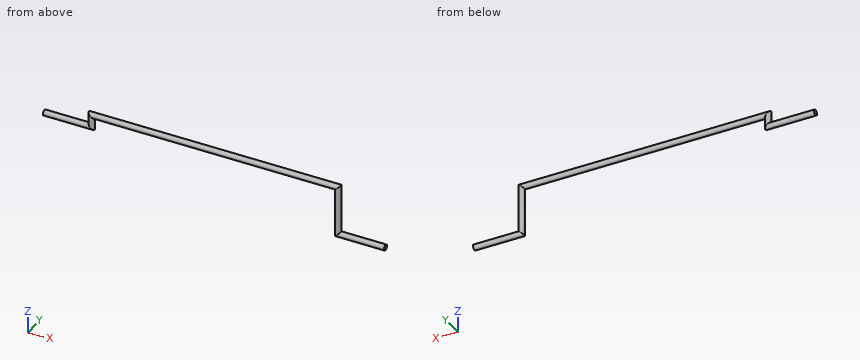
from build123d import *

# Parameters (mm, degrees)
SWEEP1_PROFILE_R = 0.6


with BuildPart() as part:
    # Sweep1: sweep along a path in Sketch1
    with BuildLine(Plane(origin=(0, 0, 0), x_dir=(1, 0, 0), z_dir=(0, 1, 0))) as sweep1_path:
        Line((62.11, 10.55), (52.11, 10.55))
        Line((52.11, 10.55), (52.11, 0))
        Line((52.11, 0), (0, 0))
        Line((0, 0), (0, 2.6))
        Line((0, 2.6), (-10, 2.6))
    # Sweep1 profile (on start of the path) → Sweep1 (sweep)
    with BuildSketch(Plane(origin=(62.11, 0, -10.55), x_dir=(0, 0, -1), z_dir=(-1, 0, 0))):
        Circle(SWEEP1_PROFILE_R)
    sweep(path=sweep1_path.line, transition=Transition.RIGHT)


solid = part.part
Check sheet for the modelled part. Datum: model origin and axes. Units: mm. Give positions to 0.01 mm unless a question says otherwise; leave off trailing zeros. Order: outer loops, then holes, each group sorted by start corner. A loop starts at its lowest first (then second) coordinate and runs counter-clockwise, first axis right, second up. Notation, with made-up numbers: (-27.75, 51.5) - (-23.75, 51.5) arc R28 ccw to (-23.75, 80.5) - close; hole circle Ø7 at (36, 61.5). An arc over 180 degrees is marked (long way). Answer as CSV lines item,"result".
1. Section check D-D (x = -5). Record the boundary of the cut face in (y, z), then the cut area to 3 significant figures.
Result sheet:
outline,"circle Ø1.2 at (0, -2.6)"
area,"1.13 mm²"
2. Section check A-A (z = -2.6). Record the boundary of the cut face in (x, y).
Result sheet:
outline,"(-10, -0.6) - (0, -0.6) arc R0.6 ccw to (0, 0.6) - (-10, 0.6) - close; circle Ø1.2 at (52.11, 0)"
3. Scan lines: probe 1 along Z at (x, y) = (39, -0.05); probe 2 along X at (y, z) = (0.4, -1.5); probe 3 along X at (y, z) = (-0.3, -1). Record each from-to range of solid material in increasing order. Write a range as from..to.
Result sheet:
probe 1,"-0.6..0.6"
probe 2,"-0.45..0.45, 51.66..52.56"
probe 3,"-0.52..0.52, 51.59..52.63"
4. Section check B-B (y = 0). Record the boundary of the cut face in (x, z), then the cut area to 3 significant figures.
Result sheet:
outline,"(-10, -3.2) - (0.6, -3.2) - (0.6, -0.6) - (51.51, -0.6) - (51.51, -11.15) - (62.11, -11.15) - (62.11, -9.95) - (52.71, -9.95) - (52.71, 0.6) - (-0.6, 0.6) - (-0.6, -2) - (-10, -2) - close"
area,"102 mm²"
5. Section check C-C (z = 0). Record the boundary of the cut face in (x, y), then the cut area to 3 significant figures.
Result sheet:
outline,"(0, -0.6) - (52.11, -0.6) arc R0.6 ccw to (52.11, 0.6) - (0, 0.6) arc R0.6 ccw to start"
area,"63.7 mm²"
